Check sheet for the drawn part. Datum: minimum x, y, z corner. Units: mm. A direction names the side the tool comes from. Coordinates: 2 decimals unless noted, no trailing zeros. Order: outer loops, then holes, each group sorted by start corner. A loop starts at its lowest first (then second) coordinate and runs counter-clockwise, first axis right, second up.
1. Cross-section at C-C (x = 24.5). Enter the section's corners in (y, z).
2. Thickness scan on line 1 (Z direction, x = 29.5, y = 19.5); line 2 (Y direction, x = 19, z = 7.5) (1 decimal); line 3 (Y direction, x = 14.5, z = 20) (1 decimal). Record the ranges inside material, lowest first.
3. Set-up check for the marked faces 1, 2, 3 and 4: record each of +Z, -Z, +X, -X, +Y, -Y from which the full face is reachable in a straight line by a thin tool's end or side.
4. Cross-section at B-B (z = 21.75). Enter the section's corners in (x, y).
5. Gauge pin test, flat ends, axial feed: pin 1 Ø3 at (y, z) = (1.5, 4.5) entering from -X (1 decimal); pin 2 Ø8 at (y, z) = (22, 16.5) entering from +X (1 decimal); pin 3 Ø1.5 at (y, z) = (23, 14) entering from +X; pin 4 Ø3 at (y, z) = (14, 4.5) entering from +X (1 decimal). Record the tip position at first contact, or that the pin passes through.
6. Cross-section at A-A (y = 19). Enter the section's corners in (x, z).
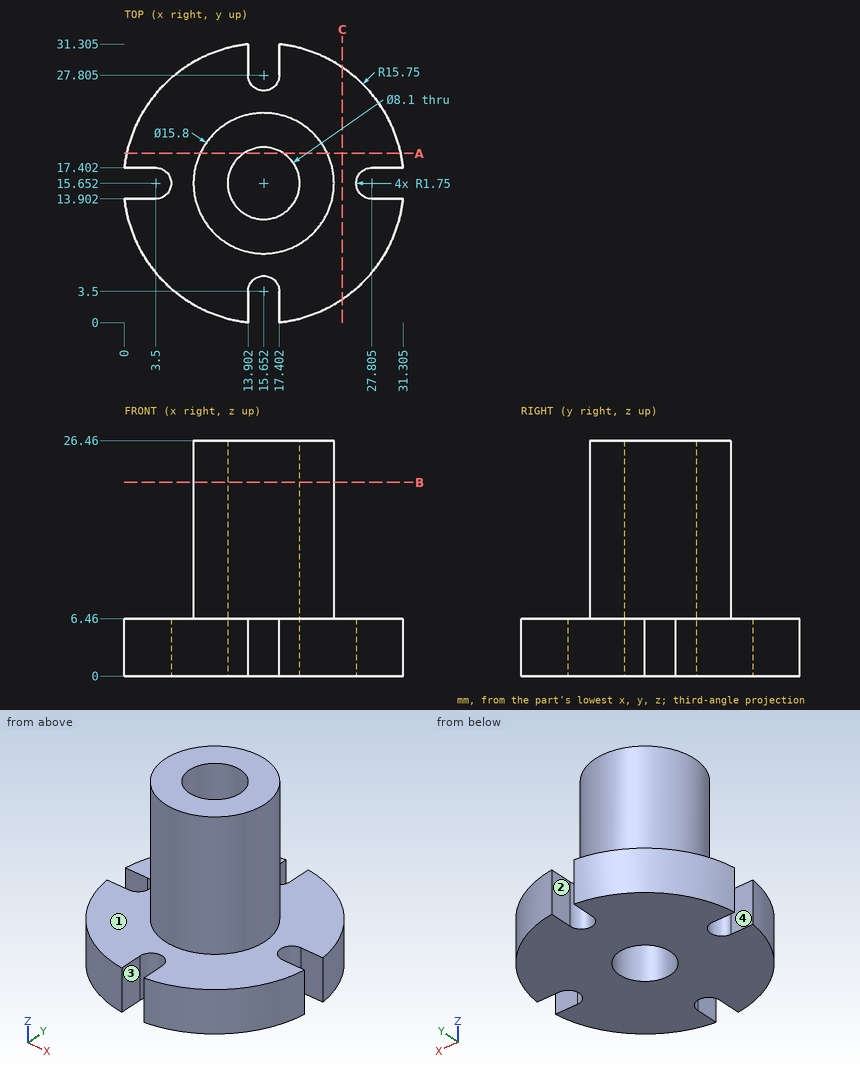
Data:
1. outline: (2.62, 0) - (28.68, 0) - (28.68, 6.46) - (2.62, 6.46) - close
2. line 1: z = 0 to 6.46
2. line 2: y = 8.5 to 13.4, 17.9 to 22.8
2. line 3: y = 7.8 to 11.8, 19.5 to 23.5
3. face 1: +Z
3. face 2: +Z, -Z, +Y
3. face 3: +Z, -Z, -Y
3. face 4: +Z, -Z, -X
4. outline: circle Ø15.8 at (15.65, 15.65); hole circle Ø8.1 at (15.65, 15.65)
5. pin 1: stops at x = 6.3
5. pin 2: stops at x = 23.2
5. pin 3: stops at x = 20
5. pin 4: stops at x = 31.3
6. outline: (0.26, 0) - (13.37, 0) - (13.37, 26.46) - (8.5, 26.46) - (8.5, 6.46) - (0.26, 6.46) - close; (17.93, 0) - (31.04, 0) - (31.04, 6.46) - (22.81, 6.46) - (22.81, 26.46) - (17.93, 26.46) - close
